```python
from build123d import *

# Parameters (mm, degrees)
F1_DEPTH = 12.7
F2_R     = 2.54
F3_W     = 9.28931
F3_H     = 14.83982
F4_DEPTH = 2.54


with BuildPart() as f1:
    # F0 (on Top) → F1 (new body)
    with BuildSketch(Plane.XY):
        with BuildLine():
            Line((96.829839, 35.876159), (-128.277585, 35.876159))
            ThreePointArc((-128.277585, 35.876159), (-146.238097, 28.436672), (-153.677585, 10.476159))
            Line((-153.677585, 10.476159), (-153.677585, -42.501916))
            ThreePointArc((-153.677585, -42.501916), (-146.238097, -60.462429), (-128.277585, -67.901916))
            Line((-128.277585, -67.901916), (96.829839, -67.901916))
            ThreePointArc((96.829839, -67.901916), (114.790351, -60.462429), (122.229839, -42.501916))
            Line((122.229839, -42.501916), (122.229839, 10.476159))
            ThreePointArc((122.229839, 10.476159), (114.790351, 28.436672), (96.829839, 35.876159))
        make_face()
        with BuildLine():
            Line((71.429839, -42.501916), (-102.877585, -42.501916))
            ThreePointArc((-102.877585, -42.501916), (-120.838097, -35.062429), (-128.277585, -17.101916))
            Line((-128.277585, -17.101916), (-128.277585, -14.923841))
            ThreePointArc((-128.277585, -14.923841), (-120.838097, 3.036672), (-102.877585, 10.476159))
            Line((-102.877585, 10.476159), (71.429839, 10.476159))
            ThreePointArc((71.429839, 10.476159), (89.390351, 3.036672), (96.829839, -14.923841))
            Line((96.829839, -14.923841), (96.829839, -17.101916))
            ThreePointArc((96.829839, -17.101916), (89.390351, -35.062429), (71.429839, -42.501916))
        make_face(mode=Mode.SUBTRACT)
    extrude(amount=F1_DEPTH)

    # F2
    f2_edges = [f1.edges().sort_by_distance(p)[0] for p in [
        (-15.723873, 35.876159, 12.7),
        (-146.238097, 28.436672, 12.7),
        (-153.677585, -16.012879, 12.7),
        (-146.238097, -60.462429, 12.7),
        (-15.723873, -67.901916, 12.7),
        (114.790351, -60.462429, 12.7),
        (122.229839, -16.012879, 12.7),
        (114.790351, 28.436672, 12.7),
        (-15.723873, -42.501916, 12.7),
        (-120.838097, -35.062429, 12.7),
        (-128.277585, -16.012879, 12.7),
        (-120.838097, 3.036672, 12.7),
        (-15.723873, 10.476159, 12.7),
        (89.390351, 3.036672, 12.7),
        (96.829839, -16.012879, 12.7),
        (89.390351, -35.062429, 12.7),
    ]]
    fillet(f2_edges, radius=F2_R)

    # F3 (on face) → F4 (join)
    with BuildSketch(Plane.XY.offset(12.7)):
        with Locations((-110.76466, -53.500641)):
            Rectangle(F3_W, F3_H)
    extrude(amount=F4_DEPTH)


solid = f1.part
```
Part model, mm, in its own coordinate system. A direction names the side the tool comes from. Coordinates: 2 decimals unless noted, no trailing zeros. Order: outer loops, then holes, each group sorted by start corner. A loop starts at its lowest first (then second) coordinate and runs counter-clockwise, first axis right, second up. Notation, with made-up numbers: (4, -29.75) -> (30, -29.75) arc R31 cw to (30, 7.25) -> close; hole circle Ø4 at (56.25, 89.25). An arc over 180 degrees is marked (long way). Put each result on its own line as item: value. Start each with the question number.
(1) Band-saw the part on A-A (x = -88). Give the cut face in (y, z).
(2) Which spindle directions (+Z, -Z, +X, -X, +Y, -Y) get a long thin tool onto all of the face, cutting with end or side? Do faces 1 (the face through (-14, 35.876, 5)), 2 (the face through (-121.03, 2.84, 5.01)). Say none if no direction does.
(3) Pin check, flat tips, straight feed: pin 1 Ø1 at (y, z) = (-52, 9) entering from +X; pin 2 Ø0.8 at (y, z) = (-52.5, 13.5) entering from +X; pin 3 Ø4 at (x, y) = (-104.5, 12.5) entering from +Z. Stop position of each tip, or through.
(4) Probe line 1 along Y through (x, z) = (-41, 3.25); line 2 along Y through (x, z) = (98, 8.5); line 3 along X through (y, z) = (-8, 1.25). List the from-to ranges inside material, lowest first. Write a range as [from, to].
(5) Mould opens along Y. For faces 3 (the face through (-153.678, -16, 5)), 4 (the face through (-146.04, 28.63, 5.01)), 5 (the face through (-120.6, -35.3, 5)) say: pulls with the +Y half, pulls with the -Y half, needs draft (parallel to the pull), parting line crosses it, or undercut.
(6) Band-saw the part on B-B (z = 6.5). Give the cut face in (x, y).
Determined:
1. outline: (-67.9, 0) -> (-42.5, 0) -> (-42.5, 10.16) arc R2.54 ccw to (-45.04, 12.7) -> (-65.36, 12.7) arc R2.54 ccw to (-67.9, 10.16) -> close; (10.48, 0) -> (35.88, 0) -> (35.88, 10.16) arc R2.54 ccw to (33.34, 12.7) -> (13.02, 12.7) arc R2.54 ccw to (10.48, 10.16) -> close
2. face 1: +Z, -Z, +X, -X, +Y
2. face 2: +Z, -Z
3. pin 1: stops at x = 120.58
3. pin 2: stops at x = -106.12
3. pin 3: stops at z = 12.7
4. line 1: y = [-67.9, -42.5], [10.48, 35.88]
4. line 2: y = [-67.87, 35.85]
4. line 3: x = [-153.68, -127.32], [95.87, 122.23]
5. face 3: needs draft
5. face 4: pulls with the +Y half
5. face 5: undercut
6. outline: (-153.68, -42.5) arc R25.4 ccw to (-128.28, -67.9) -> (96.83, -67.9) arc R25.4 ccw to (122.23, -42.5) -> (122.23, 10.48) arc R25.4 ccw to (96.83, 35.88) -> (-128.28, 35.88) arc R25.4 ccw to (-153.68, 10.48) -> close; hole (-128.28, -17.1) arc R25.4 ccw to (-102.88, -42.5) -> (71.43, -42.5) arc R25.4 ccw to (96.83, -17.1) -> (96.83, -14.92) arc R25.4 ccw to (71.43, 10.48) -> (-102.88, 10.48) arc R25.4 ccw to (-128.28, -14.92) -> close
